Geometry check sheet. Reference: the model listing, model coordinates, mm. A direction names the side the tool comes from. Round coordinates to 2 decimals unless told otherwise and drop trailing zeros. Write each loop counter-clockwise with the first axis right and the second up, starting at its lowest first coordinate (ties: lowest second). Pieces come first, ordered by that corner, then holes. Notation, with made-up numbers: M 58,44 L 82,44 A12 ccw 82,65 Z; hole C 20.25,28.5 d1. An arc over 180 degrees is marked long. One line per item, written item: value. Start each with the question number.
1. Depth check by flat-ended pin: P1, Ø2.5, axis at y = 5, z = -3.5, coming from the -X side; P2, Ø2.5, axis at y = 15.5, z = -1.5, coming from the +X side; P3, Ø0.8, axis at x = 2, y = 3, coming from the +Z side. Enter the tip coordinate at first touch or a pass-through.
2. Release check for a two-part mould opening along Y. For faces 1 (the flat face through (0, 14, -3)), 2 (the flat face through (0, 14.5, 0)), 3 (the flat face through (-0.75, 16, 0)), 4 (the flat face through (0.021, 4.816, -3.376)) record: pulls with the +Y half, pulls with the -Y half, needs draft (parallel to the pull), parting line crosses it, or undercut.
3. Section check C-C (y = 2.25). Record the boundary of the cut face in (x, z), and give its area (3 significant figures).
4. Section check A-A (y = 10.25). Record the boundary of the cut face in (x, z), and give its area (3 significant figures).
5. Access from +Z, -Z, +X, -X, +Y, -Y to the whole of each face (thin tool, end or side, straight path). Record for faces 5 (the flat face through (0.75, 16, 0)), 6 (the flat face through (0, 0, 0)), 7 (the flat face through (0, 14, 3)), 8 (the flat face through (0.021, 8.444, -2.027)), 9 (the flat face through (0, 9.5, -5)).
6. Section check D-D (y = 12). Record the boundary of the cut face in (x, z).
7. Scan lines: probe 1 along X at (y, z) = (2.8, 0); probe 2 along Z at (x, y) = (0.5, 14); probe 3 along Z at (x, y) = (-2.25, 1.2). Record each from-to range of solid material in increasing order. Write a range as [from, to].
8. Section check B-B (z = 0). Record the boundary of the cut face in (x, y), and give its area (4 significant figures).
from build123d import *

# Parameters (mm, degrees)
BOSS_EXTRUDE2_DEPTH = 1.5
BOSS_EXTRUDE3_DEPTH = 4.5
SKETCH1_3_R         = 0.63
SKETCH1_3_R_2       = 0.36
CUT_EXTRUDE2_DEPTH  = 19.862460073
BOSS_EXTRUDE4_REACH = 22.02
SKETCH3_W           = 1.5
SKETCH3_H           = 3


with BuildPart() as part:
    # Sketch2 → Boss-Extrude2 (new, symmetric)
    with BuildSketch(Plane(origin=(0, 0, 0), x_dir=(0, 0, -1), z_dir=(1, 0, 0))):
        Polygon((-6, 12.5), (-6, 9.5), (-4.5, 9.5), (-2.22, 0), (0, 0), (-3, 12.5), (-3, 17.5), (-6, 17.5), align=None)
    boss_extrude2 = extrude(amount=BOSS_EXTRUDE2_DEPTH, both=True)

    # Sketch1 → Boss-Extrude3 (add)
    with BuildSketch(Plane(origin=(0, 0, 0), x_dir=(1, 0, 0), z_dir=(0, 1, 0))):
        with BuildLine():
            Line((-2.2, 1.48), (2.2, 1.48))
            ThreePointArc((2.2, 1.48), (3.68, 0), (2.2, -1.48))
            Line((2.2, -1.48), (-2.2, -1.48))
            ThreePointArc((-2.2, -1.48), (-3.68, 0), (-2.2, 1.48))
        make_face()
    extrude(amount=BOSS_EXTRUDE3_DEPTH)

    # Mirror1: Boss-Extrude2 across plane
    add(boss_extrude2.mirror(Plane.XY))

    # Sketch1_3 → Cut-Extrude2 (cut, through all)
    with BuildSketch(Plane(origin=(0, 0, 0), x_dir=(1, 0, 0), z_dir=(0, 1, 0))):
        with Locations(Location((-2.25, 0, 0), (0, 0, 270))):
            Circle(SKETCH1_3_R)
        with Locations(Location((0.414349108, 0.541981393, 0), (0, 0, 270))):
            Circle(SKETCH1_3_R_2)
        with Locations(Location((1.451183077, -0.541981393, 0), (0, 0, 270))):
            Circle(SKETCH1_3_R_2)
    extrude(amount=CUT_EXTRUDE2_DEPTH, mode=Mode.SUBTRACT)

    # Sketch3 → Boss-Extrude4 (add, up to next)
    with BuildSketch(Plane.XY.offset(-3), mode=Mode.PRIVATE) as boss_extrude4_sk1:
        with Locations((0, 16)):
            Rectangle(SKETCH3_W, SKETCH3_H)
    boss_extrude4_tool1 = extrude(boss_extrude4_sk1.sketch, amount=BOSS_EXTRUDE4_REACH, mode=Mode.PRIVATE) - part.part
    add(boss_extrude4_tool1.solids().sort_by_distance((0, 16, -3))[0])


solid = part.part
Result sheet:
1. P1: stops at x = -1.5
1. P2: stops at x = 0.75
1. P3: stops at z = 1.48
2. face 1: undercut
2. face 2: undercut
2. face 3: needs draft
2. face 4: pulls with the -Y half
3. outline: M -2.2,-1.48 L -1.5,-1.48 L -1.5,-2.76 L 1.5,-2.76 L 1.5,-1.48 L 2.2,-1.48 A1.48 ccw 2.2,1.48 L 1.5,1.48 L 1.5,2.76 L -1.5,2.76 L -1.5,1.48 L -2.2,1.48 A1.48 ccw Z; hole C -2.25,0 d1.26; hole C 0.41,-0.54 d0.72; hole C 1.45,0.54 d0.72
3. area: 25.5 mm2
4. outline: M -1.5,-6 L 1.5,-6 L 1.5,-2.46 L -1.5,-2.46 Z; M -1.5,2.46 L 1.5,2.46 L 1.5,6 L -1.5,6 Z
4. area: 21.2 mm2
5. face 5: +X, +Y
5. face 6: +Z, -Z, +X, -X, -Y
5. face 7: none
5. face 8: +X, -X
5. face 9: -Z, +X, -X, -Y
6. outline: M -1.5,-6 L 1.5,-6 L 1.5,-2.88 L -1.5,-2.88 Z; M -1.5,2.88 L 1.5,2.88 L 1.5,6 L -1.5,6 Z
7. probe 1: x = [-3.68, -2.88], [-1.62, 3.68]
7. probe 2: z = [-6, -3], [3, 6]
7. probe 3: z = [-1.48, -0.63], [0.63, 1.48]
8. outline: M -3.68,0 L -2.88,0 L -2.88,4.5 L -3.68,4.5 Z; M -1.62,0 L 3.68,0 L 3.68,4.5 L -1.62,4.5 Z; M -0.75,14.5 L 0.75,14.5 L 0.75,17.5 L -0.75,17.5 Z
8. area: 31.95 mm2
